Work out the finished part from the listing and answer in its coordinate system (mm). Round coordinates to 2 decimals unless told otherwise and drop trailing zeros. Write each loop counter-clockwise with the first axis right and the second up, starting at its lowest first coordinate (ties: lowest second). Pieces come first, ordered by that corner, then holes.
1. Determine the mould class of faces 1 (the face through (6, 1, -35)), 2 (the face through (58, 0, -35)) for opening direction Z: pulls with the +Z half, pulls with the -Z half, needs draft (parallel to the pull), parting line crosses it, or undercut.
2. Find section A-A (z = -35). Write down the section's boundary in (x, y), and give its area (3 significant figures).
3. Straight lines are drawn through the part: probe 1 along X at (y, z) = (0.8, -36); probe 2 along X at (y, z) = (1, -33). For each, find the intervals that lie inside material, in ascending order.
Autodesk Inventor part; units mm, degrees
ref_plane "YZ Plane" through (0, 0, 0) normal (1, 0, 0) x (0, 1, 0)
ref_plane "XZ Plane" through (0, 0, 0) normal (0, 1, 0) x (-1, 0, 0)
ref_plane "XY Plane" through (0, 0, 0) normal (0, 0, 1) x (1, 0, 0)
sketch "スケッチ1" plane through (0, 0, 0) normal (0, 1, 0) x (-1, 0, 0)
  line L0 (0, 0) -> (-114, 0)
  line L1 (-114, 0) -> (-114, -70)
  line L2 (-114, -70) -> (0, -70)
  line L3 (0, -70) -> (0, 0)
  dimension "d0" = 114
  dimension "d1" = 70
extrude "押し出し1" add sketch "スケッチ1" along normal blind 1.5
sketch "スケッチ2" plane through (0, 1.5, 0) normal (0, 1, 0) x (1, 0, 0)
  line L0 (0, 70) -> (0, 0)
  circle A0 centre (0, 35) radius 6
  dimension "d4" = 12
extrude "押し出し2" cut sketch "スケッチ2" against normal blind 3
properties part number "COVER_revised"
Worked answers:
1. face 1: undercut
1. face 2: needs draft
2. outline: (6, 0) - (114, 0) - (114, 1.5) - (6, 1.5) - close
2. area: 162 mm2
3. probe 1: x = 5.92 to 114
3. probe 2: x = 5.66 to 114
